Design review of the part built by this model. Coordinates are the model's own, in mm. A direction names the side the tool comes from. Coordinates: 2 decimals unless noted, no trailing zeros. Write each loop counter-clockwise with the first axis right and the second up, starting at its lowest first coordinate (ties: lowest second). Pieces come first, ordered by that corner, then holes.
Q1. Take a section at A-A (x = -6). Give the boundary of the cut face in (y, z).
Q2. Machinability: for faces 4 (the flat face through (-19, 5.3, 5)), 5 (the flat face through (-21, 5.5, 5)), 6 (the flat face through (-26.2, -1, 5.5)), 7 (the flat face through (-30.9, -1, 5)), 8 (the flat face through (-9.388, 2.782, 5.423)), which of the approach directions +Z, -Z, +X, -X, +Y, -Y give a long, thin tool a straight path to every point of the face, cutting with its end or side? Answer none if there is none.
Q3. Mouldability with a two-part tool opening along Y and no side actions: class faces 1 (the flat face through (-27.4, -1, 5.5)), 2 (the flat face through (-20, -2.5, 5)), 3 (the flat face through (-18, -1, 11)) as pulls with the +Y half, pulls with the -Y half, needs draft (parallel to the pull), parting line crosses it, or undercut.
Q4. Insertion check: pin 1 (1.2 mm diameter, centred on x = -19, z = 4.5, fed in from +Y); pin 2 (1.5 mm diameter, centred on x = -16.5, z = 6, fed in from -Y); pin 3 (0.6 mm diameter, centred on x = -34, z = 6.5, fed in from +Y); pin 4 (1.5 mm diameter, centred on x = -28, y = -4, fed in from +Z). Each pin has a flat end and moves straight along its axis. Give the tip position at first contact, or say it passes through.
Q5. For probe 1 along Y at (x, z) = (-25.5, 2.25); probe 2 along Y at (x, z) = (-26.5, 4.5); probe 3 along X at (y, z) = (-2, 3.5), list the stretches that pass through material, from the lowest coordinate up.
Q6. Take a section at B-B (x = -19). Give the boundary of the cut face in (y, z), and give its area (3 significant figures).
```python
from build123d import *

# Parameters (mm, degrees)
BOSS_EXTRUDE1_DEPTH   = 11
BOSS_EXTRUDE1_2_DEPTH = 11
SKETCH2_W             = 5.7
SKETCH2_H             = 6
CUT_EXTRUDE1_DEPTH    = 3
BOSS_EXTRUDE8_DEPTH   = 11
BOSS_EXTRUDE2_DEPTH   = 6
BOSS_EXTRUDE3_START   = -5.5
BOSS_EXTRUDE3_DEPTH   = 2.5
FILLET7_R             = 1
FILLET8_R             = 1
FILLET10_R            = 1
FILLET11_R            = 1
FILLET12_R            = 0.5
BOSS_EXTRUDE7_REACH   = 45.115
BOSS_EXTRUDE7_START   = 5.5
SKETCH6_R             = 5.5
SKETCH6_R_2           = 4.5
CUT_EXTRUDE3_DEPTH    = 38.615023594
BOSS_EXTRUDE9_DEPTH   = 11


with BuildPart() as part:
    # Sketch1 → Boss-Extrude1 (new body)
    with BuildSketch(Plane.XY):
        Polygon((0, 3.8), (0, 2), (-18, 3.5), (-31, 3.5), (-32.5, 4), (-34, 3.5), (-35.5, 3.5), (-35.5, 5.3), (-34, 5.3), (-32.5, 5.8), (-31, 5.3), (-18, 5.3), align=None)
    extrude(amount=BOSS_EXTRUDE1_DEPTH)



with BuildPart() as body_2:
    # Sketch1 → Boss-Extrude1 2 (new body)
    with BuildSketch(Plane.XY):
        Polygon((0, 0), (0, -2.5), (-35.5, -2.5), (-35.5, 0), (-34, 0), (-32.5, -0.5), (-31, 0), align=None)
    extrude(amount=BOSS_EXTRUDE1_2_DEPTH)

    # Sketch2 → Cut-Extrude1 (cut)
    with BuildSketch(Plane.XZ.offset(2.5)):
        with Locations((-28.05, 5.5)):
            Rectangle(SKETCH2_W, SKETCH2_H)
    extrude(amount=-CUT_EXTRUDE1_DEPTH, mode=Mode.SUBTRACT)


with BuildPart() as part_1:
    add(part.part)

    add(body_2.part)  # Boss-Extrude8 merges body 2
    # Sketch8 → Boss-Extrude8 (add)
    with BuildSketch(Plane(origin=(0, 0, 0), x_dir=(-1, 0, 0), z_dir=(0, 0, -1))):
        with BuildLine():
            Line((1.013298532, 2.084441544), (0, 2))
            Line((0, 2), (0, 0))
            Line((0, 0), (1.1, 0))
            ThreePointArc((1.1, 0), (0.05687804, 1.000635709), (1.013298532, 2.084441544))
        make_face()
    extrude(amount=-BOSS_EXTRUDE8_DEPTH)

    # Sketch3 → Boss-Extrude2 (add)
    with BuildSketch(Plane.XY.offset(2.5)):
        Polygon((-25.2, 0), (-27.2, -2), (-27.2, -2.5), (-25.2, -2.5), align=None)
    extrude(amount=BOSS_EXTRUDE2_DEPTH)

    # Sketch4 → Boss-Extrude3 (add, symmetric)
    with BuildSketch(Plane.XY.offset(11).offset(BOSS_EXTRUDE3_START)):
        with BuildLine():
            Line((-28.4, -2), (-26.4, 0))
            Line((-26.4, 0), (-26.4, 0.4))
            Line((-26.4, 0.4), (-27.9, 0.4))
            Line((-27.9, 0.4), (-27.9, 1.9))
            ThreePointArc((-27.9, 1.9), (-27.43137085, 3.03137085), (-26.3, 3.5))
            Line((-26.3, 3.5), (-29.8, 3.5))
            Line((-29.8, 3.5), (-29.8, -3))
            Line((-29.8, -3), (-28.4, -3))
            Line((-28.4, -3), (-28.4, -2))
        make_face()
    extrude(amount=BOSS_EXTRUDE3_DEPTH, both=True)

    # Fillet7
    fillet7_edges = [part_1.edges().sort_by_distance(p)[0] for p in [
        (-35.5, 0, 5.5),
    ]]
    fillet(fillet7_edges, radius=FILLET7_R)

    # Fillet8
    fillet8_edges = [part_1.edges().sort_by_distance(p)[0] for p in [
        (-35.5, 3.5, 5.5),
    ]]
    fillet(fillet8_edges, radius=FILLET8_R)

    # Fillet10
    # the kernel refuses this fillet: 1 mm, written as the material it takes off along each edge
    with BuildSketch(Plane(origin=(-35.5, 5.3, -2.449489743), x_dir=(1.6076029396566988e-12, -1.0, 0), z_dir=(0, 0, 1))) as fillet10_piece_1:
        with BuildLine():
            CenterArc((1, 0.979795897), FILLET10_R, 180, 78.463040967)
            Line((0, 0.979795897), (-0.02, 0.979795897))
            Line((-0.02, 0.979795897), (-0.02, 0))
            Line((-0.02, 0), (0, -0.02))
            ThreePointArc((0, -0.02), (0.4, -0.02), (0.796, -0.019595918))
            Line((0.796, -0.019595918), (0.8, 0))
        make_face()
    extrude(amount=15.898979486, mode=Mode.SUBTRACT)

    # Fillet11
    fillet11_edges = [part_1.edges().sort_by_distance(p)[0] for p in [
        (-35.5, -2.5, 5.5),
    ]]
    fillet(fillet11_edges, radius=FILLET11_R)

    # Fillet12
    fillet12_edges = [part_1.edges().sort_by_distance(p)[0] for p in [
        (-28.4, -3, 5.5),
        (-29.8, -3, 5.5),
    ]]
    fillet(fillet12_edges, radius=FILLET12_R)

    # Sketch6 → Boss-Extrude7 (add, up to next)
    with BuildSketch(Plane(origin=(0, 0, 0), x_dir=(1, 0, 0), z_dir=(0, 1, 0)).offset(BOSS_EXTRUDE7_START), mode=Mode.PRIVATE) as boss_extrude7_sk1:
        with Locations(Location((-16, -5.5, 0), (0, 0, 270))):
            Circle(SKETCH6_R)
        with Locations(Location((-16, -5.5, 0), (0, 0, 270))):
            Circle(SKETCH6_R_2, mode=Mode.SUBTRACT)
    boss_extrude7_tool1 = extrude(boss_extrude7_sk1.sketch, amount=-BOSS_EXTRUDE7_REACH, mode=Mode.PRIVATE) - part_1.part
    add(boss_extrude7_tool1.solids().sort_by_distance((-16, 5.5, 0.155563))[0])

    # Sketch7 → Cut-Extrude3 (cut, through all)
    with BuildSketch(Plane.XY):
        Polygon((-18, 5.5), (-8, 4.666666667), (-8, 5.5), align=None)
    extrude(amount=CUT_EXTRUDE3_DEPTH, mode=Mode.SUBTRACT)

    # Sketch10 → Boss-Extrude9 (add)
    with BuildSketch(Plane(origin=(0, 0, 0), x_dir=(-1, 0, 0), z_dir=(0, 0, -1))):
        Polygon((0, -2.5), (4.936344802, -2.5), (0, -5.35), align=None)
    extrude(amount=-BOSS_EXTRUDE9_DEPTH)


solid = part_1.part
```
Response:
1. outline: (-2.5, 0) - (0, 0) - (0, 11) - (-2.5, 11) - close; (2.5, 0) - (4.3, 0) - (4.3, 11) - (2.5, 11) - close
2. face 4: +X, +Y
2. face 5: +Z, -Z, +X, +Y
2. face 6: none
2. face 7: -Y
2. face 8: +Z, -Z
3. face 1: undercut
3. face 2: pulls with the -Y half
3. face 3: needs draft
4. pin 1: stops at y = 5.3
4. pin 2: stops at y = -2.5
4. pin 3: stops at y = 5.4
4. pin 4: passes through
5. probe 1: y = -2.5 to 0, 3.5 to 5.3
5. probe 2: y = -2.5 to -1.3, -0.1 to 0.4, 3.49 to 5.3
5. probe 3: x = -35.37 to -30.9, -29.8 to -28.4, -27.2 to 0
6. outline: (-2.5, 0) - (0, 0) - (0, 11) - (-2.5, 11) - close; (3.5, 0) - (5.3, 0) - (5.3, 0.89) - (5.5, 0.89) - (5.5, 2.15) - (5.3, 2.15) - (5.3, 8.85) - (5.5, 8.85) - (5.5, 10.11) - (5.3, 10.11) - (5.3, 11) - (3.5, 11) - close
6. area: 47.8 mm2
